Source: CAD feature listing. Evaluate the final solid. Frame: model axes, mm. A direction names the side the tool comes from. Give positions to 0.01 mm unless a question says otherwise; leave off trailing zeros. Order: outer loops, then holes, each group sorted by start corner. A loop starts at its lowest first (then second) coordinate and runs counter-clockwise, first axis right, second up.
```python
from build123d import *

# Parameters (mm, degrees)
SKETCH2_R               = 20.25
BOSS_EXTRUDE1_DEPTH     = 200
SKETCH3_R               = 40
SKETCH3_R_2             = 5
SKETCH3_R_3             = 4
BOSS_EXTRUDE2_DEPTH     = 5
CUT_EXTRUDE5_DEPTH      = 6
CUT_EXTRUDE5_DEPTH_BACK = 201
SKETCH5_W               = 180
SKETCH5_H               = 80
CUT_EXTRUDE6_DEPTH      = 1601
SKETCH6_R               = 9
BOSS_EXTRUDE3_DEPTH     = 60


with BuildPart() as part:
    # Sketch2 → Boss-Extrude1 (new body)
    with BuildSketch(Plane.XY):
        Polygon((100, 0), (100, -50), (-1500, -50), (-1300, 50), (100, 50), align=None)
        Circle(SKETCH2_R, mode=Mode.SUBTRACT)
    extrude(amount=BOSS_EXTRUDE1_DEPTH)

    # Sketch3 → Boss-Extrude2 (add)
    with BuildSketch(Plane.XY.offset(200)):
        Circle(SKETCH3_R)
        Circle(SKETCH3_R_2, mode=Mode.SUBTRACT)
        with Locations((-30, 0)):
            Circle(SKETCH3_R_3, mode=Mode.SUBTRACT)
        with Locations((0, 30)):
            Circle(SKETCH3_R_3, mode=Mode.SUBTRACT)
        with Locations((30, 0)):
            Circle(SKETCH3_R_3, mode=Mode.SUBTRACT)
        with Locations((0, -30)):
            Circle(SKETCH3_R_3, mode=Mode.SUBTRACT)
    extrude(amount=BOSS_EXTRUDE2_DEPTH)

    # Sketch4 → Cut-Extrude5 (cut, two sides)
    with BuildSketch(Plane.XY.offset(200)) as cut_extrude5_sk:
        with BuildLine():
            Line((-0.95, 6.801251402), (-0.95, 12.900595285))
            ThreePointArc((-0.95, 12.900595285), (-6.767664084, 11.023909541), (-11.07399335, 6.685396773))
            Line((-11.07399335, 6.685396773), (-5.777899362, 3.711522544))
            ThreePointArc((-5.777899362, 3.711522544), (-3.701724404, 5.784181625), (-0.95, 6.801251402))
        make_face()
        with BuildLine():
            Line((6.801251402, 0.95), (12.900595285, 0.95))
            ThreePointArc((12.900595285, 0.95), (11.023909541, 6.767664084), (6.685396773, 11.07399335))
            Line((6.685396773, 11.07399335), (3.711522544, 5.777899362))
            ThreePointArc((3.711522544, 5.777899362), (5.784181625, 3.701724404), (6.801251402, 0.95))
        make_face()
        with BuildLine():
            Line((0.95, -6.801251402), (0.95, -12.900595285))
            ThreePointArc((0.95, -12.900595285), (6.767664084, -11.023909541), (11.07399335, -6.685396773))
            Line((11.07399335, -6.685396773), (5.777899362, -3.711522544))
            ThreePointArc((5.777899362, -3.711522544), (3.701724404, -5.784181625), (0.95, -6.801251402))
        make_face()
        with BuildLine():
            Line((-6.801251402, -0.95), (-12.900595285, -0.95))
            ThreePointArc((-12.900595285, -0.95), (-11.023909541, -6.767664084), (-6.685396773, -11.07399335))
            Line((-6.685396773, -11.07399335), (-3.711522544, -5.777899362))
            ThreePointArc((-3.711522544, -5.777899362), (-5.784181625, -3.701724404), (-6.801251402, -0.95))
        make_face()
    extrude(amount=CUT_EXTRUDE5_DEPTH, mode=Mode.SUBTRACT)
    extrude(cut_extrude5_sk.sketch, amount=-CUT_EXTRUDE5_DEPTH_BACK, mode=Mode.SUBTRACT)

    # Sketch5 → Cut-Extrude6 (cut, through all)
    with BuildSketch(Plane(origin=(100, 0, 0), x_dir=(0, 0, -1), z_dir=(1, 0, 0))):
        with Locations((-100, 0)):
            Rectangle(SKETCH5_W, SKETCH5_H)
    extrude(amount=-CUT_EXTRUDE6_DEPTH, mode=Mode.SUBTRACT)

    # Sketch6 → Boss-Extrude3 (add)
    with BuildSketch(Plane(origin=(0, -40, 0), x_dir=(1, 0, 0), z_dir=(0, 1, 0))):
        with Locations((-1430, -150)):
            Circle(SKETCH6_R)
        with Locations((-1430, -50)):
            Circle(SKETCH6_R)
    extrude(amount=-BOSS_EXTRUDE3_DEPTH)


solid = part.part
```
1) Section query B-B, the plane z = 118.5. Return the cut outline in (x, y), and give its area (3 significant figures).
Report:
outline: (-1500, -50) - (100, -50) - (100, -40) - (-1480, -40) - close; (-1320, 40) - (100, 40) - (100, 50) - (-1300, 50) - close
area: 30,000 mm2
2) Draft query along X for faces 1 (the cylindrical face through (11, 17, 195)), 2 (the cylindrical face through (-8.67, -39.05, 202.46)), 3 (the flat face through (-1482, -41, 92)). Return one class per face: +X half, -X half, draft (parallel to the pull), parting line (faces both ways), or undercut.
Report:
face 1: undercut
face 2: parting line
face 3: -X half
3) Reachability of faces 4 (the flat face through (4, -4, 200)), 5 (the flat face through (-600, 40, 101)), 6 (the flat face through (-610, 50, 99)) from +Z, -Z, +X, -X, +Y, -Y: full face, straight path, thin tool, end or side. Return the list, or none.
Report:
face 4: -Z
face 5: +X, -X
face 6: +Z, -Z, +X, -X, +Y
4) Section query C-C, the plane y = -70. Return the cut outline in (x, z), and give its area (3 significant figures).
Report:
outline: circle Ø18 at (-1430, 50); circle Ø18 at (-1430, 150)
area: 509 mm2
5) Material intervals for L1, parallel to Y at x = 0, z = 202; L2, parallel to Y at x = -1130, z = 131; L3, parallel to Y at x = 0, z = 198, sorted ascending.
Report:
L1: y = -40 to -34, -26 to -5, 5 to 26, 34 to 40
L2: y = -50 to -40, 40 to 50
L3: y = -50 to -20.25, 20.25 to 50
6) Section query A-A, the plane x = -479. Return the cut outline in (y, z), and give its area (3 significant figures).
Report:
outline: (-50, 0) - (50, 0) - (50, 200) - (-50, 200) - close; hole (-40, 10) - (40, 10) - (40, 190) - (-40, 190) - close
area: 5,600 mm2
7) Pin query (flat end, axial travel): pin 1 (2.5 mm diameter, centred on x = 2, y = -31, fed in from +Z); pin 2 (4 mm diameter, centred on x = -964, z = 36.5, fed in from -Y); pin 3 (2.5 mm diameter, centred on x = -10.5, z = 203.5, fed in from -Y). Return the tip coordinate at first contact, or that it passes through.
Report:
pin 1: stops at z = 200
pin 2: stops at y = -50
pin 3: stops at y = -38.92
